from build123d import *

# Parameters (mm, degrees)
CYLINDER276_R             = 10
CYLINDER276_DEPTH         = 30
CYLINDER110_R             = 3.5
CYLINDER110_DEPTH         = 30
CYLINDER109_R             = 4.7
CYLINDER109_DEPTH         = 30
FUSION080_ROLL_ANGLE      = 180
FUSION080_PLACEMENT_ANGLE = -90
CYLINDER269_R             = 1.4
CYLINDER269_DEPTH         = 50
CYLINDER268_R             = 1.4
CYLINDER268_DEPTH         = 50
CYLINDER030_R             = 1.7
CYLINDER030_DEPTH         = 19
CYLINDER030_ROLL_ANGLE    = 90
CYLINDER107_R             = 1.7
CYLINDER107_DEPTH         = 19
CYLINDER107_ROLL_ANGLE    = 90
CYLINDER108_R             = 1.7
CYLINDER108_DEPTH         = 19
CYLINDER108_ROLL_ANGLE    = 90
CYLINDER104_R             = 1.7
CYLINDER104_DEPTH         = 19
CYLINDER104_ROLL_ANGLE    = 90
BOX001012_W               = 14
BOX001012_H               = 2.8
BOX001012_DEPTH           = 11
BOX001011_W               = 14
BOX001011_H               = 2.8
BOX001011_DEPTH           = 11
BOX001010_W               = 14
BOX001010_H               = 30
BOX001010_DEPTH           = 8
CUT006_ROLL_ANGLE         = 180
CUT006_PLACEMENT_ANGLE    = -90


with BuildPart() as cylinder290:
    # Cylinder276 → Cylinder276 (new body)
    with BuildSketch(Plane(origin=(61.5, 15, -11), x_dir=(1, 0, 0), z_dir=(0, 0, 1))):
        Circle(CYLINDER276_R)
    extrude(amount=CYLINDER276_DEPTH)


with BuildPart() as cylinder116:
    # Cylinder110 → Cylinder110 (new body)
    with BuildSketch(Plane.XY.offset(-9)):
        Circle(CYLINDER110_R)
    extrude(amount=CYLINDER110_DEPTH)


with BuildPart() as bearing_nut:
    # Cylinder109 → Cylinder109 (new body)
    with BuildSketch(Plane.XY.offset(-4.5)):
        Circle(CYLINDER109_R)
    extrude(amount=CYLINDER109_DEPTH)

    # Fusion080: union Cylinder116
    add(cylinder116.part)


with BuildPart() as bearing_nut_1:
    # Fusion080 roll: moved
    add(bearing_nut.part.rotate(Axis((0, 0, 0), (1, 0, 0)), FUSION080_ROLL_ANGLE))


with BuildPart() as bearing_nut_2:
    # Fusion080 placement: moved
    add(bearing_nut_1.part.moved(Location((61.5, 14.5, 17.5))).rotate(Axis((61.5, 14.5, 17.5), (0, 0, 1)), FUSION080_PLACEMENT_ANGLE))


with BuildPart() as m3_studding026:
    # Cylinder269 → Cylinder269 (new body)
    with BuildSketch(Plane(origin=(68.5, 15, 2), x_dir=(1, 0, 0), z_dir=(0, 0, 1))):
        Circle(CYLINDER269_R)
    extrude(amount=CYLINDER269_DEPTH)


with BuildPart() as fusion112155:
    # Cylinder268 → Cylinder268 (new body)
    with BuildSketch(Plane(origin=(54.5, 15, 2), x_dir=(1, 0, 0), z_dir=(0, 0, 1))):
        Circle(CYLINDER268_R)
    extrude(amount=CYLINDER268_DEPTH)

    # Fusion112155: union m3-studding026
    add(m3_studding026.part)


with BuildPart() as cylinder030:
    # Cylinder030 → Cylinder030 (new body)
    with BuildSketch(Plane.XY):
        Circle(CYLINDER030_R)
    extrude(amount=CYLINDER030_DEPTH)


with BuildPart() as cylinder030_1:
    # Cylinder030 roll: moved
    add(cylinder030.part.rotate(Axis((0, 0, 0), (1, 0, 0)), CYLINDER030_ROLL_ANGLE))


with BuildPart() as cylinder030_2:
    # Cylinder030 placement: moved
    add(cylinder030_1.part.moved(Location((4, 24, 6))))


with BuildPart() as cylinder107:
    # Cylinder107 → Cylinder107 (new body)
    with BuildSketch(Plane.XY):
        Circle(CYLINDER107_R)
    extrude(amount=CYLINDER107_DEPTH)


with BuildPart() as cylinder107_1:
    # Cylinder107 roll: moved
    add(cylinder107.part.rotate(Axis((0, 0, 0), (1, 0, 0)), CYLINDER107_ROLL_ANGLE))


with BuildPart() as cylinder107_2:
    # Cylinder107 placement: moved
    add(cylinder107_1.part.moved(Location((4, 24, 6))))


with BuildPart() as part_mirroring013:
    # Part__Mirroring013: instance of Cylinder107
    add(cylinder107_2.part.mirror(Plane(origin=(0, 0, 0), x_dir=(1, 0, 0), z_dir=(0, 1, 0))))


with BuildPart() as cylinder108:
    # Cylinder108 → Cylinder108 (new body)
    with BuildSketch(Plane.XY):
        Circle(CYLINDER108_R)
    extrude(amount=CYLINDER108_DEPTH)


with BuildPart() as cylinder108_1:
    # Cylinder108 roll: moved
    add(cylinder108.part.rotate(Axis((0, 0, 0), (1, 0, 0)), CYLINDER108_ROLL_ANGLE))


with BuildPart() as cylinder108_2:
    # Cylinder108 placement: moved
    add(cylinder108_1.part.moved(Location((-4, 24, 6))))


with BuildPart() as part_mirroring014:
    # Part__Mirroring014: instance of Cylinder108
    add(cylinder108_2.part.mirror(Plane(origin=(0, 0, 0), x_dir=(1, 0, 0), z_dir=(0, 1, 0))))


with BuildPart() as m3_clear_a:
    # Cylinder104 → Cylinder104 (new body)
    with BuildSketch(Plane.XY):
        Circle(CYLINDER104_R)
    extrude(amount=CYLINDER104_DEPTH)


with BuildPart() as m3_clear_a_1:
    # Cylinder104 roll: moved
    add(m3_clear_a.part.rotate(Axis((0, 0, 0), (1, 0, 0)), CYLINDER104_ROLL_ANGLE))


with BuildPart() as m3_clear_a_2:
    # Cylinder104 placement: moved
    add(m3_clear_a_1.part.moved(Location((-4, 24, 6))))

    # Fusion063: union Cylinder030, Part__Mirroring013, Part__Mirroring014
    add(cylinder030_2.part)
    add(part_mirroring013.part)
    add(part_mirroring014.part)


with BuildPart() as cube051:
    # Box001012 → Box001012 (new body)
    with BuildSketch(Plane(origin=(-7, 12.2, -1), x_dir=(1, 0, 0), z_dir=(0, 0, 1))):
        with Locations((7, 1.4)):
            Rectangle(BOX001012_W, BOX001012_H)
    extrude(amount=BOX001012_DEPTH)


with BuildPart() as cube050:
    # Box001011 → Box001011 (new body)
    with BuildSketch(Plane(origin=(-7, -15, -1), x_dir=(1, 0, 0), z_dir=(0, 0, 1))):
        with Locations((7, 1.4)):
            Rectangle(BOX001011_W, BOX001011_H)
    extrude(amount=BOX001011_DEPTH)


with BuildPart() as bearing_clamp:
    # Box001010 → Box001010 (new body)
    with BuildSketch(Plane(origin=(-7, -15, -8.5), x_dir=(1, 0, 0), z_dir=(0, 0, 1))):
        with Locations((7, 15)):
            Rectangle(BOX001010_W, BOX001010_H)
    extrude(amount=BOX001010_DEPTH)

    # Fusion061: union Cube051, Cube050
    add(cube051.part)
    add(cube050.part)

    # Cut006: cut M3-clear-a
    add(m3_clear_a_2.part, mode=Mode.SUBTRACT)


with BuildPart() as bearing_clamp_1:
    # Cut006 roll: moved
    add(bearing_clamp.part.rotate(Axis((0, 0, 0), (1, 0, 0)), CUT006_ROLL_ANGLE))


with BuildPart() as bearing_clamp_2:
    # Cut006 placement: moved
    add(bearing_clamp_1.part.moved(Location((61.5, 14.5, 17.5))).rotate(Axis((61.5, 14.5, 17.5), (0, 0, 1)), CUT006_PLACEMENT_ANGLE))

    # Cut240: cut Fusion112155
    add(fusion112155.part, mode=Mode.SUBTRACT)

    # Cut241: cut bearing-nut
    add(bearing_nut_2.part, mode=Mode.SUBTRACT)

    # Cut252: cut Cylinder290
    add(cylinder290.part, mode=Mode.SUBTRACT)


solid = bearing_clamp_2.part
Geometry check sheet. Reference: the model listing, model coordinates, mm. A direction names the side the tool comes from. Round coordinates to 2 decimals unless told otherwise and drop trailing zeros. Order: outer loops, then holes, each group sorted by start corner. A loop starts at its lowest first (then second) coordinate and runs counter-clockwise, first axis right, second up. Notation, with made-up numbers: M 84,71.25 L 124,71.25 A14 ccw 124,81.25 Z; hole C 31,63.5 d5. An arc over 180 degrees is marked long. Write each question's results on one line, items separated by ' | '. Start each with the question number.
1. Cross-section at B-B on x = 61.5. Record the boundary of the cut face in (y, z), plus the area to 3 significant figures.
2. Cross-section at C-C on y = 14.5. Record the boundary of the cut face in (x, z).
3. Set-up check for faces 1 (the face through (66.09, 15.52, 20.52)), 2 (the face through (48, 15, 7.5)), 3 (the face through (73.7, 15, 13)): record each of +Z, -Z, +X, -X, +Y, -Y from which the full face is reachable in a straight line by a thin tool's end or side.
4. Material ranges on L1, parallel to Y at x = 75.4, z = 11.5; L2, parallel to X at y = 9.25, z = 17.75; L3, parallel to Z at x = 47.5, y = 10.5, recorded low to high. Write a range as from..to.
5. Cross-section at A-A on z = 17.25. Record the boundary of the cut face in (x, y).
6. Cross-section at D-D on z = 11.5. Record the boundary of the cut face in (x, y).
7. Go/stop test with a flat-tipped pin: P1, Ø3, axis at x = 68.5, y = 15, coming from the -Z side. Record where the tip stops, or that it passes through.
8. Draft check along X on faces 4 (the face through (62, 21.5, 21)), 5 (the face through (46.5, 15, 17)), 6 (the face through (55.835, 15.421, 22.451)). Enter one of: pulls with the +X half, pulls with the -X half, needs draft (parallel to the pull), parting line crosses it, or undercut.
Resolved:
1) outline: M 7.5,19 L 9.8,19 L 9.8,22 L 11,22 L 11,26 L 7.5,26 Z; M 18,22 L 19.2,22 L 19.2,19 L 21.5,19 L 21.5,26 L 18,26 Z | area: 41.8 mm2
2) outline: M 46.5,7.5 L 49.3,7.5 L 49.3,18 L 51.51,18 L 51.51,19 L 53.19,19 L 53.19,26 L 46.5,26 Z; M 55.81,19 L 56.8,19 L 56.8,22 L 58,22 L 58,26 L 55.81,26 Z; M 65,22 L 66.2,22 L 66.2,19 L 67.19,19 L 67.19,26 L 65,26 Z; M 69.81,19 L 71.49,19 L 71.49,18 L 73.7,18 L 73.7,7.5 L 76.5,7.5 L 76.5,26 L 69.81,26 Z
3) face 1: -Z | face 2: -Z, +X, -X, +Y, -Y | face 3: -Z, +Y, -Y
4) L1: 7.5..8.8, 12.2..16.8, 20.2..21.5 | L2: 46.5..49.3, 73.7..76.5 | L3: 7.5..9.8, 13.2..26
5) outline: M 46.5,7.5 L 49.3,7.5 L 49.3,21.5 L 46.5,21.5 Z; M 73.7,7.5 L 76.5,7.5 L 76.5,21.5 L 73.7,21.5 Z
6) outline: M 46.5,7.5 L 49.3,7.5 L 49.3,8.8 L 46.5,8.8 Z; M 46.5,12.2 L 49.3,12.2 L 49.3,16.8 L 46.5,16.8 Z; M 46.5,20.2 L 49.3,20.2 L 49.3,21.5 L 46.5,21.5 Z; M 73.7,7.5 L 76.5,7.5 L 76.5,8.8 L 73.7,8.8 Z; M 73.7,12.2 L 76.5,12.2 L 76.5,16.8 L 73.7,16.8 Z; M 73.7,20.2 L 76.5,20.2 L 76.5,21.5 L 73.7,21.5 Z
7) P1: z = 19
8) face 4: needs draft | face 5: pulls with the -X half | face 6: undercut
